Answer from the drawing. Dimensions are ordinates in mm from the lowest x, y and z of the part. Round coordinates to 2 decimals unless told otherwise and drop trailing zeros. Order: outer loops, then holes, each group sorted by start corner. A loop starts at its lowest first (then second) coordinate and runs counter-clockwise, first axis right, second up. Notation, with made-up numbers: (88, 47) -> (123, 47) arc R19 cw to (123, 74) -> close; hole circle Ø1 at (12, -31.5). An arc over 180 degrees is marked (long way). Use a Markdown table: item, result. Add a question column.
Item 1: For a pull along X with two mould halves and no side action, classify the marked faces 1, 2 and 3 as +X half, -X half, draft (parallel to the pull), parting line (faces both ways), or undercut.
Item 2: A cutting plane is placed at C-C, the plane z = 20.75. Determine the outline of the cut face in (x, y).
Item 3: A cutting plane is placed at D-D, the plane x = 3.25. Determine the outline of the cut face in (y, z).
Item 4: Flat-ended cylindrical pins translate along their axes: P1, Ø6.5, axis at x = 5.5, z = 23, coming from the -Y side; P2, Ø1, axis at y = 1, z = 10, coming from the +X side; P3, Ø0.6, axis at y = 1.5, z = 12.5, coming from the -X side; P4, Ø1, axis at x = 1.5, y = 1, coming from the +Z side. Find the tip coordinate at first contact, or state that the pin passes through.
Item 5: A cutting plane is placed at A-A, the plane x = 5.5. Determine the outline of the cut face in (y, z) (3 decimals), plus the area to 3 significant figures.
Item 6: Find the intervals of material crossed by L1, parallel to Z at x = 6.5, y = 1.4 (1 decimal); L2, parallel to Z at x = 5.25, y = 0.55; L3, parallel to X at y = 0.45, z = 14.75, in increasing order. Write a range as [from, to].
Item 7: A cutting plane is placed at B-B, the plane y = 1.55. Give the number of separate pieces and of enclosed holes in the cut face, plus the area to 3 significant figures.
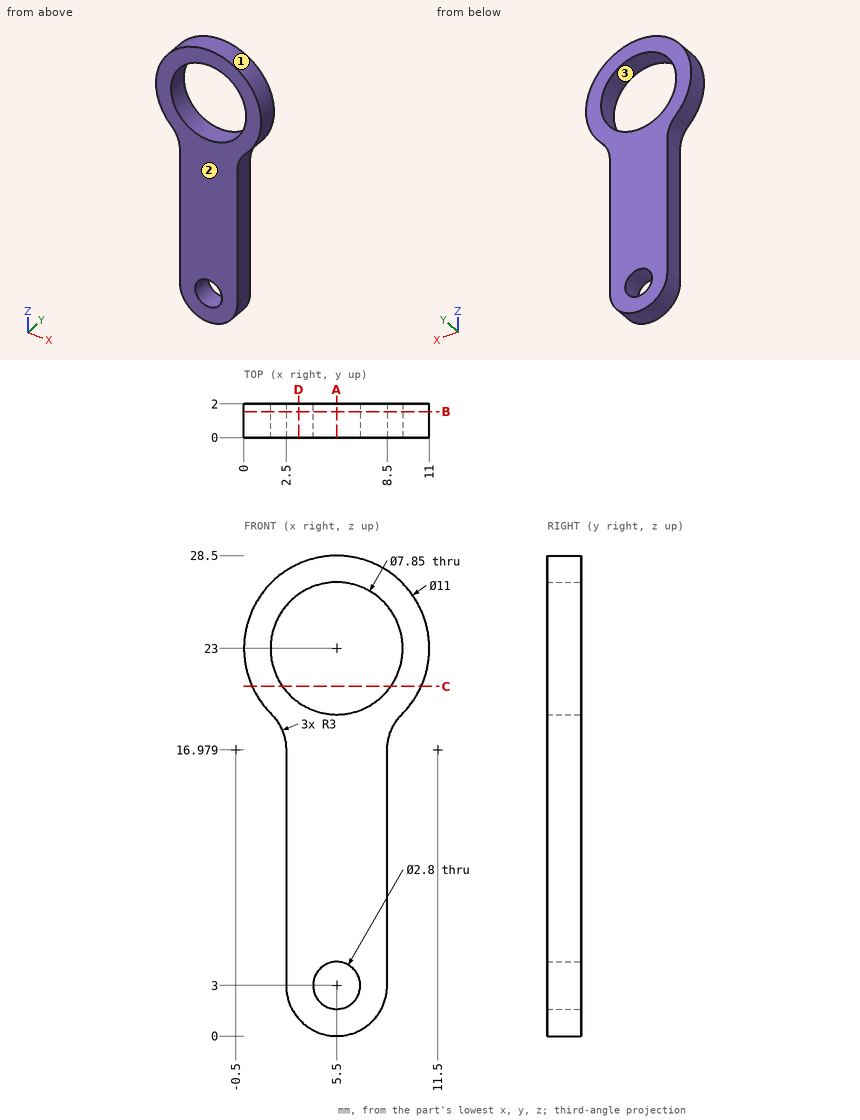
Reported:
| question | item | result |
|---|---|---|
| 1 | face 1 | parting line |
| 1 | face 2 | draft |
| 1 | face 3 | undercut |
| 2 | outline | (0.48, 0) -> (2.28, 0) -> (2.28, 2) -> (0.48, 2) -> close; (8.72, 0) -> (10.52, 0) -> (10.52, 2) -> (8.72, 2) -> close |
| 3 | outline | (0, 1.02) -> (2, 1.02) -> (2, 19.78) -> (0, 19.78) -> close; (0, 26.22) -> (2, 26.22) -> (2, 28.02) -> (0, 28.02) -> close |
| 4 | P1 | through |
| 4 | P2 | x = 8.5 |
| 4 | P3 | x = 2.5 |
| 4 | P4 | z = 27.24 |
| 5 | outline | (0, 0) -> (2, 0) -> (2, 1.6) -> (0, 1.6) -> close; (0, 4.4) -> (2, 4.4) -> (2, 19.075) -> (0, 19.075) -> close; (0, 26.925) -> (2, 26.925) -> (2, 28.5) -> (0, 28.5) -> close |
| 5 | area | 35.7 mm² |
| 6 | L1 | [0.2, 2], [4, 19.2], [26.8, 28.4] |
| 6 | L2 | [0.01, 1.62], [4.38, 19.08], [26.92, 28.49] |
| 6 | L3 | [2.5, 8.5] |
| 7 | separate pieces | 1 |
| 7 | enclosed holes | 2 |
| 7 | area | 144 mm² |
